Here's the drawing with two shaded views (mm, measured from the low corner). I have some questions. A direction names the side the tool comes from. Coordinates: 2 decimals unless noted, no trailing zeros. Write each loop counter-clockwise with the first axis right and the second up, starting at its lowest first coordinate (ties: lowest second). Pieces come first, ordered by that corner, then holes.
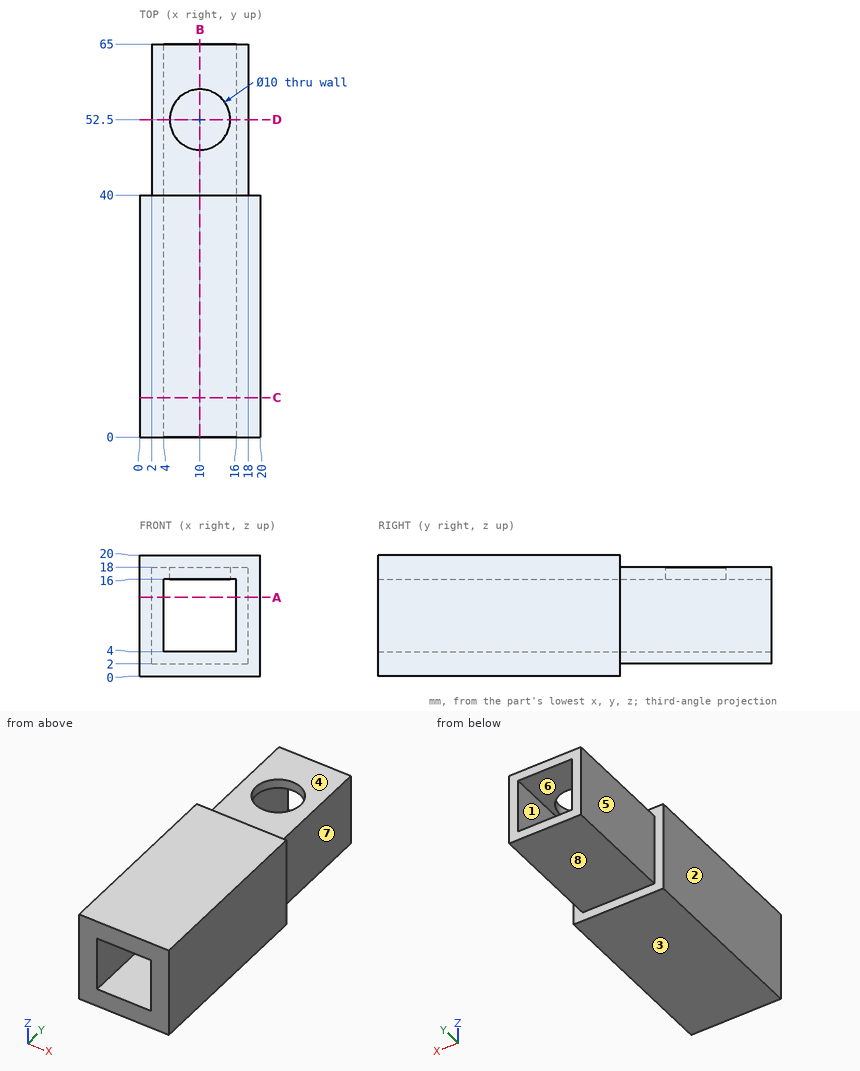
1. Please list where these lines run through material, in increasing order: line 1 along Y through (x, z) = (10, 16.7); line 2 along Z through (x, y) = (13.5, 48); line 3 along X through (y, z) = (25.5, 6.25).
Verdict:
line 1: y = 0 to 47.5, 57.5 to 65
line 2: z = 2 to 4, 16 to 18
line 3: x = 0 to 4, 16 to 20
2. If we mould it in two halves opening along X, with no side actions, what happens to the marked faces 1, 2 and 3? For each: pulls with the +X half, pulls with the -X half, needs draft (parallel to the pull), parting line crosses it, or undercut.
Verdict:
face 1: undercut
face 2: pulls with the -X half
face 3: needs draft
3. I want a section at A-A on z = 13. Please give me the cut outline in (x, y), plus the area to 3 significant figures.
Verdict:
outline: (0, 0) - (4, 0) - (4, 65) - (2, 65) - (2, 40) - (0, 40) - close; (16, 0) - (20, 0) - (20, 40) - (18, 40) - (18, 65) - (16, 65) - close
area: 420 mm2
4. I want a section at B-B on x = 10. Please give me the cut outline in (y, z), plus the area to 3 significant figures.
Verdict:
outline: (0, 0) - (40, 0) - (40, 2) - (65, 2) - (65, 4) - (0, 4) - close; (0, 16) - (47.5, 16) - (47.5, 18) - (40, 18) - (40, 20) - (0, 20) - close; (57.5, 16) - (65, 16) - (65, 18) - (57.5, 18) - close
area: 400 mm2
5. I want a section at D-D on y = 52.5. Please give me the cut outline in (x, z).
Verdict:
outline: (2, 2) - (18, 2) - (18, 18) - (15, 18) - (15, 16) - (16, 16) - (16, 4) - (4, 4) - (4, 16) - (5, 16) - (5, 18) - (2, 18) - close
6. For pin 1 (6 mm diameter, centred on x = 10, y = 43.5, fed in from +Z); pin 2 (5 mm diameter, centred on x = 5, y = 17, fed in from -Z); pin 3 (8 mm diameter, centred on x = 8.5, y = 50, fed in from -Z); pin 4 (2 mm diameter, centred on y = 56, z = 14, fed in from -X), each with a flat end and sliding along its axis, tell me the tip position at first contact or that it passes through.
Verdict:
pin 1: stops at z = 18
pin 2: stops at z = 0
pin 3: stops at z = 2
pin 4: stops at x = 2
7. I want a section at C-C on y = 6.5. Please give me the cut outline in (x, z).
Verdict:
outline: (0, 0) - (20, 0) - (20, 20) - (0, 20) - close; hole (4, 4) - (16, 4) - (16, 16) - (4, 16) - close
8. On a 3-axis mill with a long thin cutter (end or side, diameter ignored), from which of +Z, -Z, +X, -X, +Y, -Y can I reach the whole of each face in a straight line? I mean the marked faces 4, 5, 6, 7 and 8. Say none if no direction works.
Verdict:
face 4: +Z, +X, -X, +Y
face 5: +Z, -Z, -X, +Y
face 6: +Y, -Y
face 7: +Z, -Z, +X, +Y
face 8: -Z, +X, -X, +Y
